Could you check a few things on this model? Use its own coordinates, in mm. Face numbers are marked on the shaded views. A direction names the side the tool comes from. Round coordinates to 2 decimals unless told otherwise and drop trailing zeros. Order: outer loops, then holes, each group sorted by start corner. A loop starts at its lowest first (then second) coordinate and runs counter-clockwise, first axis right, second up. Notation, with made-up numbers: (-38, -19.75) -> (14, -19.75) arc R25 cw to (14, -1.75) -> close; hole circle Ø6 at (-17, -23.5). An arc over 180 degrees is marked (long way). One line per question, with ' | ' between items.
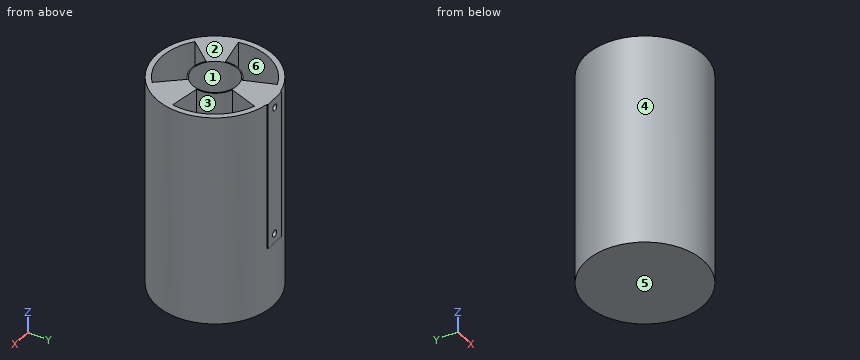
Autodesk Inventor part; units mm, degrees
ref_plane "YZ Plane" through (0, 0, 0) normal (1, 0, 0) x (0, 1, 0)
ref_plane "XZ Plane" through (0, 0, 0) normal (0, 1, 0) x (-1, 0, 0)
ref_plane "XY Plane" through (0, 0, 0) normal (0, 0, 1) x (1, 0, 0)
sketch "スケッチ1" plane through (0, 0, 0) normal (0, 0, 1) x (1, 0, 0)
  circle A0 centre (0, 0) radius 27.5
  dimension "d0" = 55
extrude "押し出し1" add sketch "スケッチ1" along normal blind 100
sketch "スケッチ2" plane through (0, 0, 100) normal (0, 0, 1) x (1, 0, 0)
  circle A0 centre (0, 0) radius 27.5
  circle A1 centre (0, 0) radius 25
  dimension "d3" = 50
extrude "押し出し2" cut sketch "スケッチ2" against normal blind 97 contours A1
sketch "スケッチ3" plane through (0, 0, 3) normal (0, 0, 1) x (1, 0, 0)
  circle A0 centre (0, 0) radius 25
  circle A1 centre (0, 0) radius 10.5
  circle A2 centre (0, 0) radius 11
  dimension "d6" = 21
  dimension "d7" = 22
extrude "押し出し3" add sketch "スケッチ3" along normal blind 97 contours A2
sketch "スケッチ4" plane through (0, 0, 100) normal (0, 0, 1) x (1, 0, 0)
  circle A0 centre (0, 0) radius 25
  circle A1 centre (0, 0) radius 27.5
  circle A2 centre (0, 0) radius 11
  line L0 (0, 0) -> (0, 25)
  line L1 (0, 0) -> (8.5505, 23.4923)
  line L2 (0, 0) -> (25, 0) construction
  line L3 (0, 0) -> (-8.5505, 23.4923)
  line L4 (0, 0) -> (25, 0) construction
  line L5 (0, 0) -> (-21.6506, -12.5)
  line L6 (0, 0) -> (25, 0) construction
  line L7 (0, 0) -> (21.6506, -12.5)
  line L8 (0, 0) -> (25, 0) construction
  line L9 (0, 0) -> (-16.0697, -19.1511)
  line L10 (0, 0) -> (25, 0) construction
  line L11 (0, 0) -> (-24.6202, -4.3412)
  line L12 (0, 0) -> (25, 0) construction
  line L13 (0, 0) -> (24.6202, -4.3412)
  line L14 (0, 0) -> (25, 0) construction
  line L15 (0, 0) -> (16.0697, -19.1511)
  line L16 (0, 0) -> (25, 0) construction
  dimension "d10" = 22
  dimension "d11" = 70
  dimension "d12" = 110
  dimension "d13" = 150
  dimension "d14" = 30
  dimension "d15" = 130
  dimension "d16" = 170
  dimension "d17" = 10
  dimension "d18" = 50
extrude "押し出し4" add sketch "スケッチ4" against normal blind 15 contours L1 A2 L0 A0 | A0 L7 A2 L13 | L0 A2 L3 A0 | L1 L0 A2 | A0 L15 A2 L7 | A2 L7 L13 | L0 L3 A2 | L9 A2 L5 | L5 A2 L11 | L7 A2 L15 | L11 A2 L5 A0 | A2 L9 A0 L5
sketch "スケッチ5" plane through (0, 0, 100) normal (0, 0, 1) x (1, 0, 0)
  arc A0 (-6.7493, -8.0435) -> (6.7493, -8.0435) centre (0, 0) ccw
  line L0 (-6.7493, -8.0435) -> (0, 0)
  line L1 (0, 0) -> (-10.3405, -1.8233)
  arc A1 (-3.5912, 9.8668) -> (-10.3405, -1.8233) centre (0, 0) ccw
  line L2 (-3.5912, 9.8668) -> (0, 0)
  line L3 (0, 0) -> (3.5912, 9.8668)
  arc A2 (10.3405, -1.8233) -> (3.5912, 9.8668) centre (0, 0) ccw
  line L4 (10.3405, -1.8233) -> (0, 0)
  line L5 (0, 0) -> (6.7493, -8.0435)
  circle A3 centre (0, 0) radius 27.5
  circle A4 centre (0, 0) radius 10.5
extrude "押し出し5" cut sketch "スケッチ5" against normal blind 15 contours A4 L1 L0 | L5 L4 A4 | L2 A4 L3
sketch "スケッチ6" plane through (0, 0, 100) normal (0, 0, 1) x (1, 0, 0)
  circle A0 centre (0, 0) radius 27.5
  line L0 (24.6202, -4.3412) -> (10.8329, -1.9101)
  arc A1 (10.8329, -1.9101) -> (3.7622, 10.3366) centre (0, 0) ccw
  line L1 (3.7622, 10.3366) -> (8.5505, 23.4923)
  arc A2 (24.6202, -4.3412) -> (8.5505, 23.4923) centre (0, 0) ccw
  arc A3 (-8.5505, 23.4923) -> (-24.6202, -4.3412) centre (0, 0) ccw
  line L2 (-8.5505, 23.4923) -> (-3.7622, 10.3366)
  arc A4 (-3.7622, 10.3366) -> (-10.8329, -1.9101) centre (0, 0) ccw
  line L3 (-10.8329, -1.9101) -> (-24.6202, -4.3412)
  arc A5 (-16.0697, -19.1511) -> (16.0697, -19.1511) centre (0, 0) ccw
  line L4 (-16.0697, -19.1511) -> (-7.0707, -8.4265)
  arc A6 (-7.0707, -8.4265) -> (7.0707, -8.4265) centre (0, 0) ccw
  line L5 (7.0707, -8.4265) -> (16.0697, -19.1511)
  circle A7 centre (0, 0) radius 10.5
  point P0 (0, 27.5)
ref_plane "作業平面1" through (0, 27.5, 100) normal (0, 1, 0) x (-1, 0, 0)
sketch "スケッチ8" plane through (0, 27.5, 100) normal (0, 1, 0) x (-1, 0, 0)
  line L0 (-4.8637, 0) -> (5.1363, 0)
  line L1 (5.1363, 0) -> (5.1363, -70)
  line L2 (5.1363, -70) -> (-4.8637, -70)
  line L3 (-4.8637, -70) -> (-4.8637, 0)
  line L4 (27.5, 0) -> (-27.5, 0)
  line L5 (0, 0) -> (0, -6)
  line L6 (0.1363, -70) -> (0.1363, -64)
  point P0 (0, -100)
  dimension "d27" = 10
  dimension "d28" = 70
  dimension "d29" = 0
  dimension "d30" = 6
  dimension "d31" = 6
extrude "押し出し6" add sketch "スケッチ8" against normal blind 1
sketch "スケッチ9" plane through (0, 27.5, 100) normal (0, 1, 0) x (1, 0, 0)
  line L0 (4.8637, 0) -> (-5.1363, 0)
  line L1 (-5.1363, 0) -> (-5.1363, 70)
  line L2 (0, 70) -> (0, 65.5)
  line L3 (-0.1363, 0) -> (-0.1363, 4.5)
  point P0 (0, 100)
  dimension "d34" = 4.5
  dimension "d35" = 4.5
hole "穴1" at (0, 27.5, 34.5) at (-0.1363, 27.5, 95.5) direction (0, -1, 0) diameter 3 depth 8 tip angle 118
thread "ねじ1"
thread "ねじ2"
sketch "スケッチ10" plane through (0, 27.5, 100) normal (0, 1, 0) x (1, 0, 0)
  circle A0 centre (0, 65.5) radius 1.5
  circle A1 centre (-0.1363, 4.5) radius 1.5
  line L0 (4.8637, 0) -> (-5.1363, 0)
  line L1 (4.8637, 70) -> (4.8637, 0)
  line L2 (0, 70) -> (4.8637, 70)
  line L3 (-5.1363, 70) -> (0, 70)
  line L4 (-5.1363, 0) -> (-5.1363, 70)
  point P0 (0, 100)
properties part number "知能ロボコンシリンダ" material "ABS プラスチック"
1. I want a section at D-D on y = 15. List the corners of the cut face in (x, z) for me, and give its area (3 significant figures).
From the geometry:
outline: (-23.05, 0) -> (23.05, 0) -> (23.05, 100) -> (20, 100) -> (20, 3) -> (-20, 3) -> (-20, 100) -> (-23.05, 100) -> close; (-5.46, 85) -> (5.46, 85) -> (5.46, 100) -> (-5.46, 100) -> close | area: 894 mm²
2. I need wall thicknesses on probe 1 along Y at (x, z) = (0, 53); probe 2 along Z at (x, y) = (-3, 22); probe 3 along X at (y, z) = (6.5, 57.5). Which ranges of each line are inside material? Lowest first, please.
From the geometry:
probe 1: y = -27.5 to -25, -11 to -10.5, 10.5 to 11, 25 to 27.5 | probe 2: z = 0 to 3, 85 to 100 | probe 3: x = -26.72 to -24.14, -8.87 to -8.25, 8.25 to 8.87, 24.14 to 26.72
3. I want a section at C-C on y = 0. List the corners of the cut face in (x, z) for me, and give its area (3 significant figures).
From the geometry:
outline: (-27.5, 0) -> (27.5, 0) -> (27.5, 100) -> (25, 100) -> (25, 3) -> (11, 3) -> (11, 100) -> (10.5, 100) -> (10.5, 3) -> (-10.5, 3) -> (-10.5, 100) -> (-11, 100) -> (-11, 3) -> (-25, 3) -> (-25, 100) -> (-27.5, 100) -> close | area: 747 mm²
4. I want a section at A-A on z = 34.5. List the corners of the cut face in (x, y) for me.
From the geometry:
outline: circle Ø22 at (0, 0); (-5.14, 27.02) arc R27.5 ccw (long way) to (4.86, 27.07) -> (4.86, 27.5) -> (1.5, 27.5) -> (1.5, 24.95) arc R25 cw (long way) to (-1.5, 24.95) -> (-1.5, 27.5) -> (-5.14, 27.5) -> close; hole circle Ø21 at (0, 0)
5. If we mould it in two halves opening along X, with no side actions, what happens to the marked faces 4, 5 and 6? For each: pulls with the +X half, pulls with the -X half, needs draft (parallel to the pull), parting line crosses it, or undercut.
From the geometry:
face 4: parting line crosses it | face 5: needs draft | face 6: undercut
6. On a 3-axis mill with a long thin cutter (end or side, diameter ignored), from which of +Z, -Z, +X, -X, +Y, -Y can I reach the whole of each face in a straight line? I mean the marked faces 1, 2 and 3. Say none if no direction works.
From the geometry:
face 1: +Z | face 2: +Z, +X, -X, +Y, -Y | face 3: none
7. I'm going to push flat-ended pins straight in: pin 1 (12 mm diameter, centred on x = 12.5, z = 28.5, fed in from +Y); pin 2 (1 mm diameter, centred on y = 20, z = 76.5, fed in from +X); pin 3 (1.5 mm diameter, centred on x = -8.5, y = -1.5, fed in from +Z). Where does each tip first touch, or does it pass through?
From the geometry:
pin 1: stops at y = 26.72 | pin 2: stops at x = 19.39 | pin 3: stops at z = 3
8. I want a section at B-B on z = 58.5. List the corners of the cut face in (x, y) for me.
From the geometry:
outline: circle Ø22 at (0, 0); (-5.14, 27.02) arc R27.5 ccw (long way) to (4.86, 27.07) -> (4.86, 27.5) -> (-5.14, 27.5) -> close; hole circle Ø50 at (0, 0); hole circle Ø21 at (0, 0)
